Can you work these out from the drawing? Everything is in mm from the part's minimum corner. A direction names the side the tool comes from. Round coordinates to 2 decimals unless told otherwise and drop trailing zeros. Loops run counter-clockwise (first coordinate to the right, second up) from the corner with the lowest first, then second, coordinate; pieces in that order, holes last. Notation, with made-up numbers: (60.5, 57.5) -> (71.5, 57.5) arc R33 ccw to (71.5, 93.5) -> close; hole circle Ø1 at (60, 54). An arc over 180 degrees is marked (long way). One line per item, written item: value.
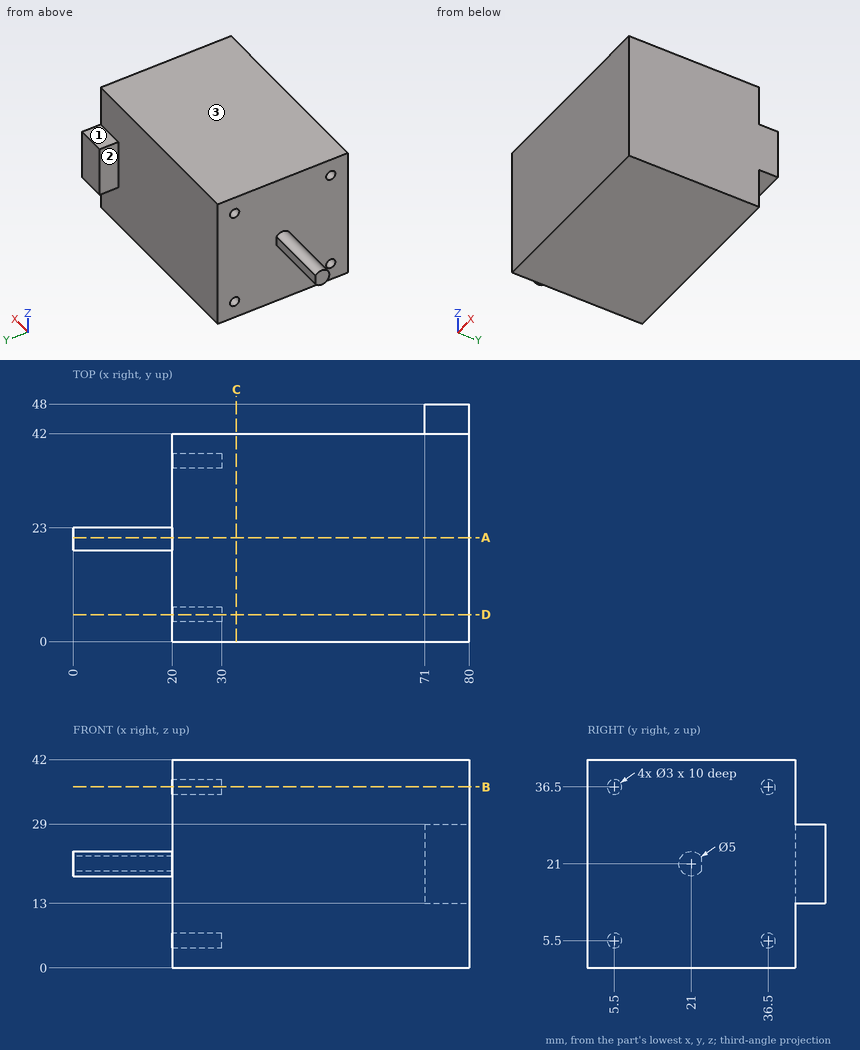
(1) On a 3-axis mill with a long thin cutter (end or side, diameter ignored), from which of +Z, -Z, +X, -X, +Y, -Y can I reach the whole of each face in a straight line? I mean the marked faces 1, 2 and 3. Say none if no direction works.
Results below:
face 1: +Z, +X, -X, +Y
face 2: +Z, -Z, -X, +Y
face 3: +Z, +X, -X, +Y, -Y
(2) Imagine slicing it at B-B on z = 36.5. Write out the boundary of the cut face in (x, y).
Results below:
outline: (20, 0) -> (80, 0) -> (80, 42) -> (20, 42) -> (20, 38) -> (30, 38) -> (30, 35) -> (20, 35) -> (20, 7) -> (30, 7) -> (30, 4) -> (20, 4) -> close
(3) For pin 1 Ø2 at (y, z) = (5.5, 34) entering from -X; pin 2 Ø0.9 at (y, z) = (5.5, 5.5) entering from -X; pin 3 Ø2.5 at (x, z) = (15, 21.5) entering from +Y, each with a flat end and sliding along its axis, tell me the tip position at first contact or that it passes through.
Results below:
pin 1: stops at x = 20
pin 2: stops at x = 30
pin 3: stops at y = 23
(4) Imagine slicing it at C-C on x = 33. Write out the boundary of the cut face in (y, z).
Results below:
outline: (0, 0) -> (42, 0) -> (42, 42) -> (0, 42) -> close
(5) Please list where these lines run through material, in increasing order: L1, parallel to Y at x = 26.5, z = 5.5; L2, parallel to Y at x = 27, z = 5.
Results below:
L1: y = 0 to 4, 7 to 35, 38 to 42
L2: y = 0 to 4.09, 6.91 to 35.09, 37.91 to 42
(6) Imagine slicing it at A-A on y = 21. Write out the boundary of the cut face in (x, z).
Results below:
outline: (0, 18.5) -> (20, 18.5) -> (20, 0) -> (80, 0) -> (80, 42) -> (20, 42) -> (20, 23.5) -> (0, 23.5) -> close
